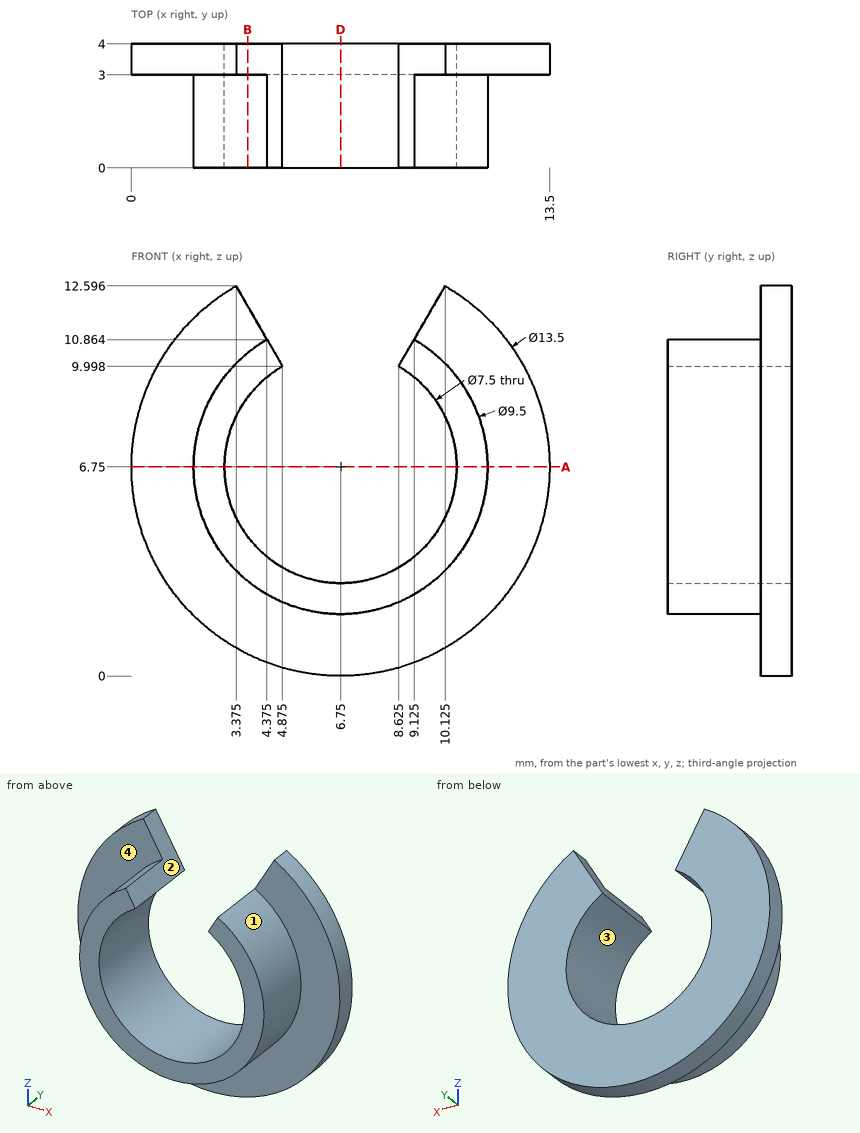
Study the drawing (mm; zero at the part's minimum x, y, z) and answer. Round coordinates to 2 decimals unless told otherwise and drop trailing zeros. Loops run counter-clockwise (first coordinate to the right, second up) from the corner with the lowest first, then second, coordinate; pieces in that order, holes last. Notation, with made-up numbers: (-16.75, 48) - (-12.75, 48) arc R21 ccw to (-12.75, 53) - close; hole circle Ø7 at (21, 32). An arc over 180 degrees is marked (long way). Use one line per item in the form item = value. Start each with the question number.
1. The part is cut by section B-B on x = 3.75. Determine the outline of the cut face in (y, z).
2. Given pin 1 Ø1.5 at (y, z) = (2, 7.5) entering from +X; pin 2 Ø2 at (x, z) = (6.5, 8) entering from +Y; pin 3 Ø4 at (x, z) = (4.5, 5.5) entering from -Y, each flat-ended and moving along its own axis, determine where each tip first touches the part or whether it passes through.
3. The part is cut by section D-D on x = 6.75. Determine the outline of the cut face in (y, z).
4. Consider line 1 (Z direction, x = 6.75, y = 2.1); line 2 (Z direction, x = 6.75, y = 3.1); line 3 (Y direction, x = 10.75, z = 11.75). Determine where each line is inside the solid, lowest interval first. Write a range as [from, to].
5. For a pull along X with two mould halves and no side action, classify the marked faces 1, 2, 3 and 4 as pulls with the +X half, pulls with the -X half, needs draft (parallel to the pull), parting line crosses it, or undercut.
6. The part is cut by section A-A on z = 6.75. Determine the outline of the cut face in (x, y).
Geometry check:
q1.outline = (0, 3.07) - (3, 3.07) - (3, 0.7) - (4, 0.7) - (4, 4.5) - (0, 4.5) - close; (0, 9) - (4, 9) - (4, 11.95) - (3, 11.95) - (3, 10.43) - (0, 10.43) - close
q2.pin_1 = 11.5
q2.pin_2 = through
q2.pin_3 = 0
q3.outline = (0, 2) - (3, 2) - (3, 0) - (4, 0) - (4, 3) - (0, 3) - close
q4.line_1 = [2, 3]
q4.line_2 = [0, 3]
q4.line_3 = [3, 4]
q5.face_1 = parting line crosses it
q5.face_2 = undercut
q5.face_3 = undercut
q5.face_4 = needs draft
q6.outline = (0, 3) - (2, 3) - (2, 0) - (3, 0) - (3, 4) - (0, 4) - close; (10.5, 0) - (11.5, 0) - (11.5, 3) - (13.5, 3) - (13.5, 4) - (10.5, 4) - close
